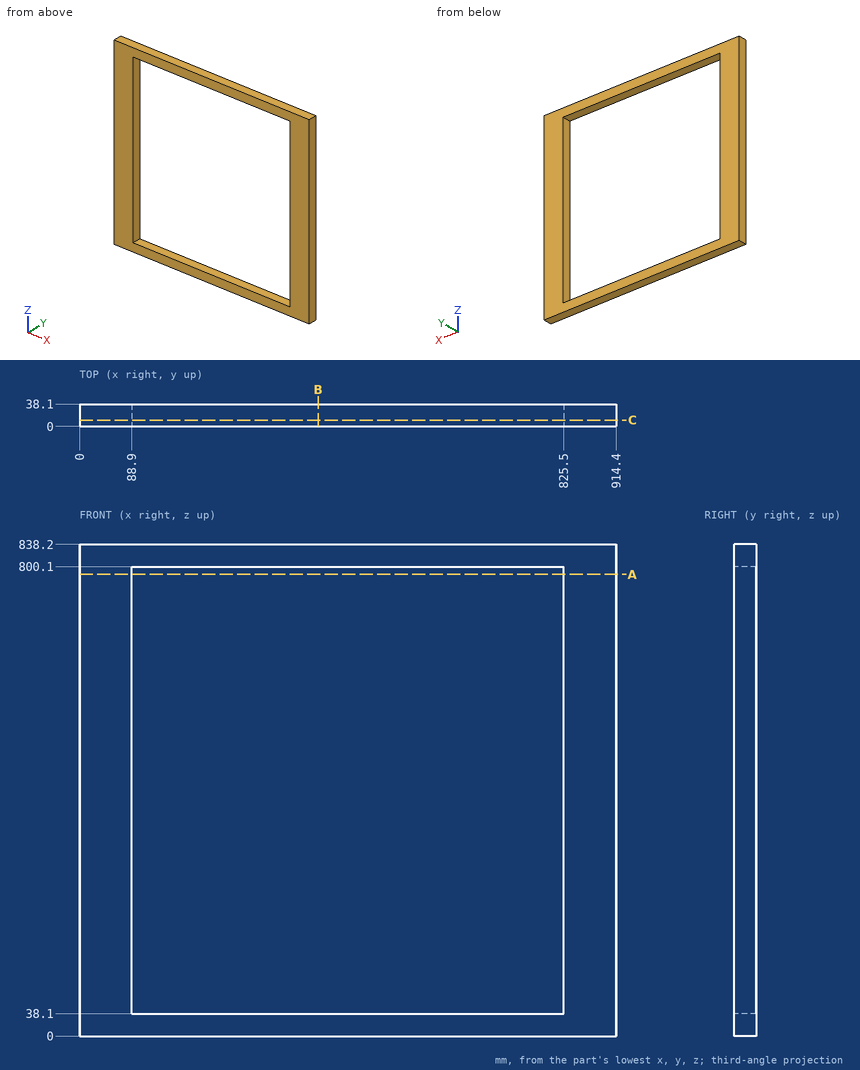
Check sheet for the drawn part. Datum: minimum x, y, z corner. Units: mm. Give positions to 0.01 mm unless a question says otherwise; leave off trailing zeros. Write each loop counter-clockwise with the first axis right and the second up, starting at its lowest first coordinate (ties: lowest second). Pieces come first, ordered by that corner, then holes.
(1) Cross-section at C-C (y = 10.5). Enter the section's corners in (x, z), plus the area to 3 significant figures.
(2) Cross-section at A-A (z = 787). Enter the section's corners in (x, y), plus the area to 3 significant figures.
(3) Material ranges on line 1 (X direction, y = 33, z = 548.5); line 2 (Z direction, x = 817, y = 29), recorded low to high.
(4) Cross-section at B-B (x = 406.5). Enter the section's corners in (y, z).
Worked out:
1. outline: (0, 0) - (914.4, 0) - (914.4, 838.2) - (0, 838.2) - close; hole (88.9, 38.1) - (825.5, 38.1) - (825.5, 800.1) - (88.9, 800.1) - close
1. area: 205,000 mm2
2. outline: (0, 0) - (88.9, 0) - (88.9, 38.1) - (0, 38.1) - close; (825.5, 0) - (914.4, 0) - (914.4, 38.1) - (825.5, 38.1) - close
2. area: 6,770 mm2
3. line 1: x = 0 to 88.9, 825.5 to 914.4
3. line 2: z = 0 to 38.1, 800.1 to 838.2
4. outline: (0, 0) - (38.1, 0) - (38.1, 38.1) - (0, 38.1) - close; (0, 800.1) - (38.1, 800.1) - (38.1, 838.2) - (0, 838.2) - close
